```python
from build123d import *

# Parameters (mm, degrees)
F1_DEPTH = 5
F2_D     = 7
F3_D     = 2


with BuildPart() as f1:
    # F0 (on Front) → F1 (new body)
    with BuildSketch(Plane.XZ):
        with BuildLine():
            ThreePointArc((0, 56), (-33, 23), (0, -10))
            ThreePointArc((0, -10), (10, 0), (0, 10))
            ThreePointArc((0, 10), (-20, 30), (0, 50))
            ThreePointArc((0, 50), (3, 53), (0, 56))
        make_face()
    extrude(amount=F1_DEPTH)

    # F2 (through all)
    with Locations(Plane(origin=(0, 0, 0), x_dir=(1, 0, 0), z_dir=(0, 1, 0))):
        with Locations((0, 0)):
            Hole(F2_D / 2)

    # F3 (through all)
    with Locations(Plane(origin=(0, 0, 0), x_dir=(1, 0, 0), z_dir=(0, 1, 0))):
        with Locations((0, 7.5), (7.5, 0), (0, -7.5), (-7.5, 0)):
            Hole(F3_D / 2)


solid = f1.part
```
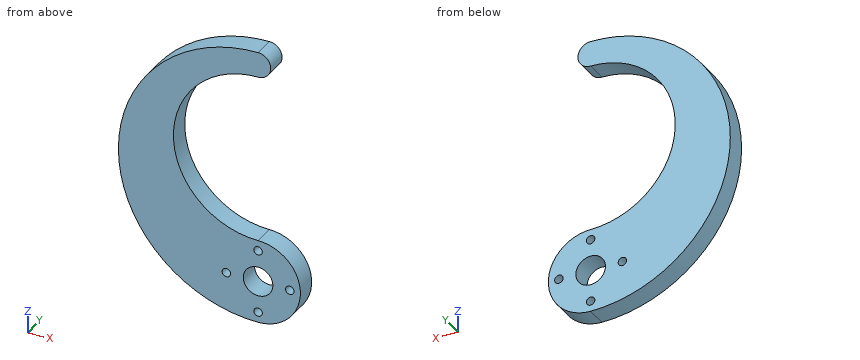
Part model, mm, in its own coordinate system. Round coordinates to 2 decimals unless told otherwise and drop trailing zeros. Order: outer loops, then holes, each group sorted by start corner. A loop starts at its lowest first (then second) coordinate and runs counter-clockwise, first axis right, second up. Notation, with made-up numbers: M -21,22.5 L -8,22.5 A19 cw -8,38.5 Z; hole C 51.25,79.25 d9. An arc over 180 degrees is marked long. Put each result on its own line as item: value. Start each with the question number.
1. Drop flat-ended pins along their axis: pin 1 (1.2 mm diameter, centred on x = -7.5, z = 0, fed in from -Y); pin 2 (1 mm diameter, centred on y = -3.5, z = 15, fed in from -X); pin 3 (2 mm diameter, centred on x = -7, y = -3.5, fed in from +Z). Give the stop position or say it passes through.
2. Slice it at C-C on z = 7.5. List the corners of the cut face in (x, y), then the cut area to 3 significant figures.
3. Slice it at A-A on y = -2.85. List the corners of the cut face in (x, z), then the cut area to 3 significant figures.
4. Drill centre lines: probe 1 along Z at (x, y) = (-7.5, -3.35); probe 2 along Z at (x, y) = (-3, -4.35); probe 3 along Z at (x, y) = (7.5, -3). Where is each one in solid material? Low to high. Write a range as [from, to].
5. Slice it at D-D on x = -26.5. List the corners of the cut face in (y, z).
6. Slice it at B-B on x = -4.5. List the corners of the cut face in (y, z), then the cut area to 3 significant figures.
Findings:
1. pin 1: through
1. pin 2: x = -32.14
1. pin 3: z = 55.45
2. outline: M -29.13,-5 L -1,-5 L -1,0 L -29.13,0 Z; M 1,-5 L 6.61,-5 L 6.61,0 L 1,0 Z
2. area: 169 mm2
3. outline: M 0,-10 A10 ccw 0,10 A20 cw 0,50 A3 ccw 0,56 A33 ccw Z; hole C -7.5,0 d2; hole C 0,0 d7; hole C 0,-7.5 d2; hole C 0,7.5 d2; hole C 7.5,0 d2
3. area: 1,200 mm2
4. probe 1: [-9.14, -1], [1, 11.46], [48.54, 55.14]
4. probe 2: [-9.86, -1.8], [1.8, 10.23], [49.77, 55.86]
4. probe 3: [-6.61, -1], [1, 6.61]
5. outline: M -5,3.33 L 0,3.33 L 0,42.67 L -5,42.67 Z
6. outline: M -5,-9.69 L 0,-9.69 L 0,10.51 L -5,10.51 Z; M -5,49.49 L 0,49.49 L 0,55.69 L -5,55.69 Z
6. area: 132 mm2
